CAD build for the part. Positions are in the model's coordinates, mm. Face numbers are marked on the shaded views. A direction names the side the tool comes from. Round coordinates to 2 decimals unless told otherwise and drop trailing zeros. Order: outer loops, then holes, each group sorted by start corner. A loop starts at its lowest first (then second) coordinate and runs counter-clockwise, first axis right, second up. Notation, with made-up numbers: M 82.25,15 L 120.25,15 A27 cw 120.25,45 Z; hole C 50.5,-21 d1. An arc over 180 degrees is marked long. Put each result on its own line as item: value.
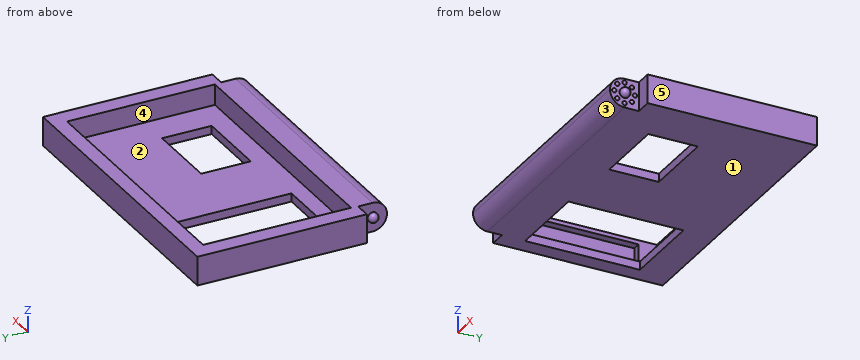
```python
from build123d import *
from build123d.topology import SkipClean

# Parameters (mm, degrees)
SKETCH_1_W               = 35.5
SKETCH_1_H               = 24
EXTRUDE_1_DEPTH          = 3.5
SKETCH_2_W               = 31.3
SKETCH_2_H               = 17.9
CUT_EXTRUDE_1_DEPTH      = 2.5
SKETCH_12_W              = 3.5
SKETCH_12_H              = 3.5
CUT_EXTRUDE_9_DEPTH      = 2
SKETCH_13_W              = 3.5
SKETCH_13_H              = 3.5
CUT_EXTRUDE_10_DEPTH     = 2
SKETCH_14_W              = 10
SKETCH_14_H              = 13.9
CUT_EXTRUDE_11_DEPTH     = 2
SKETCH_18_W              = 2
SKETCH_18_H              = 13.5
CUT_EXTRUDE_12_DEPTH     = 1
SKETCH_19_W              = 9
SKETCH_19_H              = 6
CUT_EXTRUDE_13_DEPTH     = 2
SKETCH_20_R              = 0.6
EXTRUDE_3_DEPTH          = 0.1
EXTRUDE_START            = 0.1
SKETCH_21_R              = 0.6
EXTRUDE_4_DEPTH          = 0.1
FILLET_1_R               = 1.75
FILLET_2_R               = 1.75
PATTERN_CIRCULAR_2_COUNT = 8


with BuildPart() as part:
    # 草图1 → 凸台-拉伸1 (new body)
    with BuildSketch(Plane.XY):
        Rectangle(SKETCH_1_W, SKETCH_1_H)
    extrude(amount=EXTRUDE_1_DEPTH)

    # 草图2 → 切除-拉伸1 (cut)
    with BuildSketch(Plane.XY.offset(3.5)):
        with Locations((0, 1.25)):
            Rectangle(SKETCH_2_W, SKETCH_2_H)
    extrude(amount=-CUT_EXTRUDE_1_DEPTH, mode=Mode.SUBTRACT)

    # 草图12 → 切除-拉伸9 (cut)
    with BuildSketch(Plane.ZY.offset(17.75)):
        with Locations((1.75, -10.25)):
            Rectangle(SKETCH_12_W, SKETCH_12_H)
    extrude(amount=-CUT_EXTRUDE_9_DEPTH, mode=Mode.SUBTRACT)

    # 草图13 → 切除-拉伸10 (cut)
    with BuildSketch(Plane(origin=(17.75, 0, 0), x_dir=(0, 0, -1), z_dir=(1, 0, 0))):
        with Locations((-1.75, -10.25)):
            Rectangle(SKETCH_13_W, SKETCH_13_H)
    extrude(amount=-CUT_EXTRUDE_10_DEPTH, mode=Mode.SUBTRACT)

    # 草图14 → 切除-拉伸11 (cut)
    with BuildSketch(Plane.XY.offset(1)):
        with Locations((-10.75, 1.25)):
            Rectangle(SKETCH_14_W, SKETCH_14_H)
    extrude(amount=-CUT_EXTRUDE_11_DEPTH, mode=Mode.SUBTRACT)

    # 草图18 → 切除-拉伸12 (cut)
    with BuildSketch(Plane(origin=(-15.65, 0, 0), x_dir=(0, 0, -1), z_dir=(1, 0, 0))):
        with Locations((-2, 1.25)):
            Rectangle(SKETCH_18_W, SKETCH_18_H)
    extrude(amount=-CUT_EXTRUDE_12_DEPTH, mode=Mode.SUBTRACT)

    # 草图19 → 切除-拉伸13 (cut)
    with BuildSketch(Plane.XY.offset(1)):
        with Locations((7.15, -2.2)):
            Rectangle(SKETCH_19_W, SKETCH_19_H)
    extrude(amount=-CUT_EXTRUDE_13_DEPTH, mode=Mode.SUBTRACT)

    # 草图20 → 凸台-拉伸3 (add)
    with BuildSketch(Plane.ZY.offset(15.75)):
        with Locations(Location((1.75, -10.25, 0), (0, 0, 180))):
            Circle(SKETCH_20_R)
    extrude(amount=EXTRUDE_3_DEPTH)

    # 草图21 → 凸台-拉伸4 (add)
    with BuildSketch(Plane(origin=(15.75, 0, 0), x_dir=(0, 0, -1), z_dir=(1, 0, 0)).offset(EXTRUDE_START)):
        with Locations((-1.75, -10.25)):
            Circle(SKETCH_21_R)
    extrude(amount=-EXTRUDE_4_DEPTH)

    # 草图23 → 旋转1 (revolve)
    with BuildSketch(Plane.ZY.offset(15.85)):
        with BuildLine():
            Line((1.75, -9.65), (1.75, -10.85))
            ThreePointArc((1.75, -10.85), (2.35, -10.25), (1.75, -9.65))
        make_face()
    revolve(axis=Axis((-15.85, -9.65, 1.75), (0, -1, 0)))

    # 草图24 → 旋转2 (revolve)
    with SkipClean():  # the faces are left unmerged after this step: merging them gives an invalid solid
        with BuildSketch(Plane(origin=(15.85, 0, 0), x_dir=(0, 0, -1), z_dir=(1, 0, 0))):
            with BuildLine():
                ThreePointArc((-2.140499307, -9.794467025), (-2.205532975, -10.640499307), (-1.359500693, -10.705532975))
                Line((-1.359500693, -10.705532975), (-2.140499307, -9.794467025))
            make_face()
            with BuildLine():
                Line((-2.140499307, -9.794467025), (-1.359500693, -10.705532975))
                ThreePointArc((-1.359500693, -10.705532975), (-1.204885524, -10.500699438), (-1.15, -10.25))
                ThreePointArc((-1.15, -10.25), (-1.499300562, -9.704885524), (-2.140499307, -9.794467025))
            make_face()
        revolve(axis=Axis((15.85, -10.705532975, 1.359500693), (0, 0.7592216255630779, 0.65083217750612)))
    add(part.part.scale(1), mode=Mode.REPLACE)  # the faces are merged on a copy

    # 圆角1
    fillet_1_edges = [part.edges().sort_by_distance(p)[0] for p in [
        (0, -12, 3.5),
    ]]
    fillet(fillet_1_edges, radius=FILLET_1_R)

    # 圆角2
    fillet_2_edges = [part.edges().sort_by_distance(p)[0] for p in [
        (0, -12, 0),
    ]]
    fillet(fillet_2_edges, radius=FILLET_2_R - 0.0001)  # a hair under: the kernel refuses the full size

    # 草图25 → 旋转3 (revolve)
    with BuildSketch(Plane(origin=(15.75, 0, 0), x_dir=(0, 0, -1), z_dir=(1, 0, 0))):
        with BuildLine():
            Line((-2, -9), (-1.5, -9))
            ThreePointArc((-1.5, -9), (-1.75, -8.75), (-2, -9))
        make_face()
    revolve_3 = revolve(axis=Axis((15.75, -9, 2), (0, 0, -1)))

    # 阵列(圆周)2: 旋转3 ×8 about axis
    pattern_circular_2_axis = Axis((0, -10.25, 1.75), (1, 0, 0))
    for i in range(1, PATTERN_CIRCULAR_2_COUNT):
        add(revolve_3.rotate(pattern_circular_2_axis, i * 360 / PATTERN_CIRCULAR_2_COUNT))


solid = part.part
```
Item 1: Mould opens along Y. For the marked faces 1, 2 and 3 say: pulls with the +Y half, pulls with the -Y half, needs draft (parallel to the pull), parting line crosses it, or undercut.
Answers below:
face 1: needs draft
face 2: undercut
face 3: pulls with the -Y half
Item 2: Band-saw the part on C-C on y = 2.25. Give the cut face in (x, z), and give its area (3 significant figures).
Answers below:
outline: M -17.75,0 L -15.75,0 L -15.75,1 L -16.65,1 L -16.65,3 L -15.65,3 L -15.65,3.5 L -17.75,3.5 Z; M -5.75,0 L 17.75,0 L 17.75,3.5 L 15.65,3.5 L 15.65,1 L -5.75,1 Z
area: 34.0 mm²
Item 3: Probe line 1 along Y through (x, z) = (12.5, 1.7); line 2 along Y through (x, z) = (-4, 2.65); line 3 along X through (y, z) = (1.5, 2.1). List the from-to ranges inside material, lowest first. Write a range as [from, to].
Answers below:
line 1: [-12, -7.7], [10.2, 12]
line 2: [-11.75, -7.7], [10.2, 12]
line 3: [-17.75, -16.65], [15.65, 17.75]
Item 4: Band-saw the part on A-A on y = -1.25. Give the cut face in (x, z), and give its area (3 significant figures).
Answers below:
outline: M -17.75,0 L -15.75,0 L -15.75,1 L -16.65,1 L -16.65,3 L -15.65,3 L -15.65,3.5 L -17.75,3.5 Z; M -5.75,0 L 2.65,0 L 2.65,1 L -5.75,1 Z; M 11.65,0 L 17.75,0 L 17.75,3.5 L 15.65,3.5 L 15.65,1 L 11.65,1 Z
area: 25.0 mm²
Item 5: Pin check, flat tips, straight feed: P1, Ø6, axis at x = 7, y = -2, coming from the +Z side; P2, Ø2, axis at x = -16.5, z = 2.5, coming from the -Y side; P3, Ø1.1, axis at x = -11.5, z = 0.5, coming from the -Y side. Stop position of each tip, or through.
Answers below:
P1: z = 1
P2: y = -12
P3: y = -11.85
Item 6: Tool access for the marked faces 4 and 5: list every direction of +Z, -Z, +X, -X, +Y, -Y with a clear straight run to the whole face (end or side of a thin tool).
Answers below:
face 4: +Z
face 5: +Z, -Z, +X, +Y, -Y
